Verification items for the finished model (mm, model axes). A direction names the side the tool comes from. Coordinates: 2 decimals unless noted, no trailing zeros. Write each loop counter-clockwise with the first axis right and the second up, starting at its lowest first coordinate (ties: lowest second). Pieces come first, ordered by that corner, then holes. Notation, with made-up numbers: (-23, 78.25) -> (9, 78.25) arc R26 cw to (9, 105.25) -> close; hole circle Ø3 at (43, -18.75). An arc over 180 degrees is marked (long way). Write item = value, one per line. Start each with the question number.
(1) Set-up check for faces 1 (the face through (-15, 25, 5)), 2 (the face through (-15.21, 12.325, 17.395)): record each of +Z, -Z, +X, -X, +Y, -Y from which the full face is reachable in a straight line by a thin tool's end or side.
(2) Section check C-C (z = 13.75). Record the cut outline in (x, y).
(3) Section check A-A (y = 1.5). Record the cut outline in (x, z), plus the area to 3 significant figures.
(4) Material ranges on probe 1 along Z at (x, y) = (-23, 9.5); probe 2 along X at (y, z) = (17.25, 22.5); probe 3 along Y at (x, z) = (-3.5, 14), recorded low to high. Write a range as [from, to].
(5) Gauge pin test, flat ends, axial feed: pin 1 Ø5 at (x, z) = (-25.5, 21.5) entering from +Y; pin 2 Ø1 at (y, z) = (14, 12.5) entering from -X; pin 3 Ø2 at (x, z) = (-7, 22) entering from +Y. Record the tip position at first contact, or that the pin passes through.
(6) Section check B-B (x = -27). Record the cut outline in (y, z).
```python
from build123d import *

# Parameters (mm, degrees)
SKETCH1_W           = 30
SKETCH1_H           = 25
BOSS_EXTRUDE1_DEPTH = 10
BOSS_EXTRUDE2_DEPTH = 15


with BuildPart() as part:
    # Sketch1 → Boss-Extrude1 (new body)
    with BuildSketch(Plane.XY):
        with Locations((-15, 12.5)):
            Rectangle(SKETCH1_W, SKETCH1_H)
    extrude(amount=BOSS_EXTRUDE1_DEPTH)

    # Sketch2 → Boss-Extrude2 (add)
    with BuildSketch(Plane.XY.offset(10)):
        Polygon((-30, 0), (0, 25), (0, 0), align=None)
    extrude(amount=BOSS_EXTRUDE2_DEPTH)


solid = part.part
```
Response:
q1.face_1 = +Z, -Z, +X, -X, +Y
q1.face_2 = +Z, -X, +Y
q2.outline = (-30, 0) -> (0, 0) -> (0, 25) -> close
q3.outline = (-30, 0) -> (0, 0) -> (0, 25) -> (-28.2, 25) -> (-28.2, 10) -> (-30, 10) -> close
q3.area = 723 mm2
q4.probe_1 = [0, 10]
q4.probe_2 = [-9.3, 0]
q4.probe_3 = [0, 22.08]
q5.pin_1 = 5.83
q5.pin_2 = -13.8
q5.pin_3 = 20
q6.outline = (0, 0) -> (25, 0) -> (25, 10) -> (2.5, 10) -> (2.5, 25) -> (0, 25) -> close
